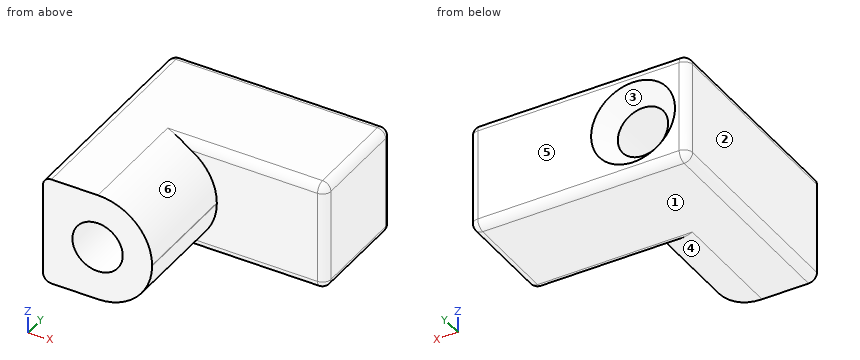
from build123d import *

# Parameters (mm, degrees)
PAD_DEPTH    = 13
SKETCH001_R  = 3
POCKET_DEPTH = 26.001
CHAMFER_SIZE = 2
FILLET_R     = 6.45
FILLET001_R  = 1
FILLET002_R  = 1
FILLET003_R  = 1


with BuildPart() as part:
    # Sketch → Pad (new body)
    with BuildSketch(Plane.XY):
        Polygon((-13, 6.5), (-13, -19.5), (0, -19.5), (0, -6.5), (13, -6.5), (13, 6.5), align=None)
    extrude(amount=PAD_DEPTH)

    # Sketch001 (on Face2 of Pad) → Pocket (cut, through all)
    with BuildSketch(Plane.XZ.offset(19.5)):
        with Locations((-6.5, 6.5)):
            Circle(SKETCH001_R)
    extrude(amount=-POCKET_DEPTH, mode=Mode.SUBTRACT)

    # Chamfer
    chamfer_edges = [part.edges().sort_by_distance(p)[0] for p in [
        (-9.5, 6.5, 6.5),
    ]]
    chamfer(chamfer_edges, length=CHAMFER_SIZE)

    # Fillet
    fillet_edges = [part.edges().sort_by_distance(p)[0] for p in [
        (0, -13, 13),
        (0, -13, 0),
    ]]
    fillet(fillet_edges, radius=FILLET_R)

    # Fillet001
    fillet001_edges = [part.edges().sort_by_distance(p)[0] for p in [
        (-13, -6.5, 13),
        (-13, -6.5, 0),
        (13, 0, 13),
        (13, 0, 0),
    ]]
    fillet(fillet001_edges, radius=FILLET001_R)

    # Fillet002
    fillet002_edges = [part.edges().sort_by_distance(p)[0] for p in [
        (0, 6.5, 0),
        (0, 6.5, 13),
        (13, 6.5, 6.5),
        (12.707107, 6.5, 0.292893),
        (12.707107, 6.5, 12.707107),
    ]]
    fillet(fillet002_edges, radius=FILLET002_R)

    # Fillet003
    fillet003_edges = [part.edges().sort_by_distance(p)[0] for p in [
        (6, -6.5, 13),
        (13, -6.5, 6.5),
        (6, -6.5, 0),
    ]]
    fillet(fillet003_edges, radius=FILLET003_R)


solid = part.part
Geometry: final body of the model. Coordinates: model frame, mm. Face numbers are marked on the shaded views. A direction names the side the tool comes from. Coordinates: 2 decimals unless noted, no trailing zeros. Loops run counter-clockwise (first coordinate to the right, second up) from the corner with the lowest first, then second, coordinate; pieces in that order, holes last. Notation, with made-up numbers: (-40, -2) - (18, -2) arc R23 ccw to (18, 37) - close; hole circle Ø9 at (71.25, -33.75). An arc over 180 degrees is marked (long way). One line per question, with ' | ' between items. Start each with the question number.
(1) Draft query along Z for the marked faces 1, 2 and 3. Return one class per face: +Z half, -Z half, draft (parallel to the pull), parting line (faces both ways), or undercut.
(2) Ray query, L1, parallel to Z at x = -6.5, y = -6.25; L2, parallel to Y at x = 11.5, z = 2.5; L3, parallel to X at y = -10.5, z = 5.25. Return the intervals inside material, ascending. Write a range as from..to.
(3) Cut plane A-A on y = -16.5. Output: boundary loops of the cut face in (x, z).
(4) Cut plane B-B on x = 2.5. Output: boundary loops of the cut face in (y, z).
(5) Reachability of the marked faces 4, 5 and 6 from +Z, -Z, +X, -X, +Y, -Y: full face, straight path, thin tool, end or side. Return the list, or none.
Here are the results:
1) face 1: -Z half | face 2: draft | face 3: undercut
2) L1: 0..3.5, 9.5..13 | L2: -6.5..6.5 | L3: -13..-9.23, -3.77..-0.11
3) outline: (-13, 1) arc R1 ccw to (-12, 0) - (-6.45, 0) arc R6.45 ccw to (0, 6.45) - (0, 6.55) arc R6.45 ccw to (-6.45, 13) - (-12, 13) arc R1 ccw to (-13, 12) - close; hole circle Ø6 at (-6.5, 6.5)
4) outline: (-6.5, 1) arc R1 ccw to (-5.5, 0) - (5.5, 0) arc R1 ccw to (6.5, 1) - (6.5, 12) arc R1 ccw to (5.5, 13) - (-5.5, 13) arc R1 ccw to (-6.5, 12) - close
5) face 4: -Z, +X, -Y | face 5: +Z, -Z, +X, -X, +Y | face 6: +Z, +X, -Y
